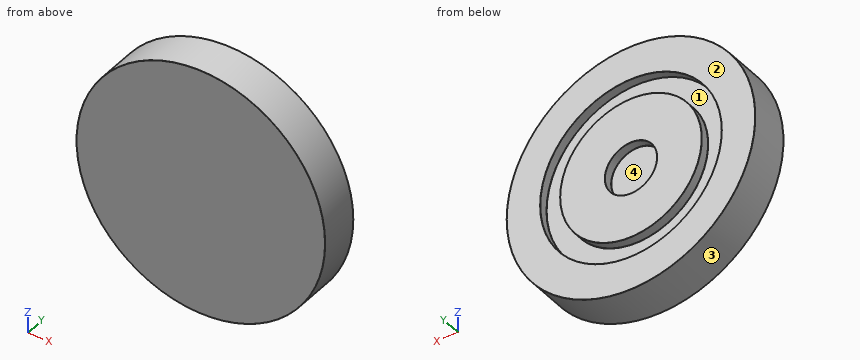
from build123d import *

# Parameters (mm, degrees)
F0_R     = 150
F1_DEPTH = 49
F2_R     = 109.5
F2_R_2   = 85.5
F2_R_3   = 31.5
F3_DEPTH = 11
F4_SIZE  = 0.1


# Not quite as in the source:
# - a feature names something its author has since deleted; it is built from what else it names


with BuildPart() as f1:
    # F0 (on Front) → F1 (new body)
    with BuildSketch(Plane.XZ):
        Circle(F0_R)
    extrude(amount=F1_DEPTH)

    # F2 (on Front) → F3 (cut)
    with BuildSketch(Plane.XZ):
        Circle(F2_R)
        Circle(F2_R_2, mode=Mode.SUBTRACT)
        Circle(F2_R_3)
    extrude(amount=F3_DEPTH, mode=Mode.SUBTRACT)

    # F4
    f4_edges = [f1.edges().sort_by_distance(p)[0] for p in [
        (-150, 0, 0),
        (150, -24.5, 0),
        (-150, -49, 0),
        (-109.5, 0, 0),
        (109.5, -5.5, 0),
        (-109.5, -11, 0),
        (-85.5, -11, 0),
        (-85.5, 0, 0),
        (85.5, -5.5, 0),
        (31.5, -5.5, 0),
        (-31.5, 0, 0),
        (-31.5, -11, 0),
    ]]
    chamfer(f4_edges, length=F4_SIZE)


solid = f1.part
Build history of the part. All positions in model axes, mm. Face numbers are marked on the shaded views. Round coordinates to 2 decimals unless told otherwise and drop trailing zeros. Write each loop counter-clockwise with the first axis right and the second up, starting at its lowest first coordinate (ties: lowest second). Pieces come first, ordered by that corner, then holes. Notation, with made-up numbers: M -13,63.25 L 37,63.25 A19 ccw 37,97.25 Z; hole C 8,-37.75 d1. An arc over 180 degrees is marked long. Answer as a JSON object with one key per item and string values. Group by question number.
(1) Cut at C-C (y = -4). Give the cut face in (x, z).
(2) Drill centre lines: L1, parallel to Z at x = 0, y = -5; L2, parallel to Z at x = 77, y = -9.5; L3, parallel to X at y = -3, z = -54.5. Where is each one in solid material? Low to high.
(3) Flat gauge pins, fed straight in: pin 1 (1.5 mm diameter, centred on x = 38, y = -18.5, fed in from -Z); pin 2 (5 mm diameter, centred on x = 99, y = -5.5, fed in from +Z); pin 3 (1 mm diameter, centred on x = 62, y = -36, fed in from -Z). Where does each tip first touch, or does it go through?
(4) Mould opens along Z. For the marked faces 1, 2, 3 and 4 say: pulls with the +Z half, pulls with the -Z half, needs draft (parallel to the pull), parting line crosses it, or undercut.
Responses:
{
 "1": {"outline": "C 0,0 d300; C 0,0 d171; hole C 0,0 d219; hole C 0,0 d63"},
 "2": {"L1": "z = -150 to -109.5, -85.5 to -31.5, 31.5 to 85.5, 109.5 to 150", "L2": "z = -128.73 to -77.85, -37.17 to 37.17, 77.85 to 128.73", "L3": "x = -139.75 to -94.97, -65.88 to 65.88, 94.97 to 139.75"},
 "3": {"pin 1": "stops at z = -145.3", "pin 2": "stops at z = 114.84", "pin 3": "stops at z = -136.81"},
 "4": {"face 1": "undercut", "face 2": "needs draft", "face 3": "parting line crosses it", "face 4": "undercut"}
}
